Geometry check sheet. Reference: the model listing, model coordinates, mm. A direction names the side the tool comes from. Round coordinates to 2 decimals unless told otherwise and drop trailing zeros. Loops run counter-clockwise (first coordinate to the right, second up) from the corner with the lowest first, then second, coordinate; pieces in that order, holes last.
Autodesk Fusion 360 part; units mm, degrees
sketch "Sketch1" plane through (0, 0, 0) normal (0, 1, 0) x (1, 0, 0)
  line L0 (0, 0) -> (20.5, 0)
  line L1 (20.5, 0) -> (20.5, -10)
  line L2 (20.5, -10) -> (0, -10)
  line L3 (0, -10) -> (0, 0)
  line L4 (25.25, 0) -> (-4.75, 0)
  line L5 (-4.75, 0) -> (-4.75, -10)
  line L6 (-4.75, -10) -> (25.25, -10)
  line L7 (25.25, -10) -> (25.25, 0)
  line L8 (25.25, 0) -> (-4.75, -10) construction
  line L9 (-4.75, 0) -> (25.25, -10) construction
  line L10 (-4.75, 0) -> (-4.75, 6)
  line L11 (-4.75, 6) -> (25.25, 6)
  line L12 (25.25, 0) -> (25.25, 6)
  line L13 (-4.75, 6) -> (-4.75, 10)
  line L14 (-4.75, 10) -> (25.25, 10)
  line L15 (25.25, 10) -> (25.25, 6)
  line L16 (10.25, 0) -> (10.25, 10) construction
  line L17 (10.25, 0) -> (10.25, 2) construction
  line L18 (10.25, 2) -> (17.25, 2) construction
  line L19 (17.25, 2) -> (10.25, 2) construction
  line L20 (10.25, 2) -> (3.25, 2) construction
  circle A0 centre (3.25, 4) radius 2
  circle A1 centre (17.25, 4) radius 2
  point P0 (10.25, -5)
  dimension "d1" = 20.5
  dimension "d2" = 10
  dimension "d3" = 30
  dimension "d4" = 10
  dimension "d5" = 6
  dimension "d6" = 2
  dimension "d7" = 7
  dimension "d8" = 7
  dimension "d9" = 4
extrude "Extrude1" add sketch "Sketch1" along normal blind 40 contours L0 L4 L10 L11 L12 | L3 L4 L5 L6 | L1 L4 L6 L7 | L11 L13 L14 L15
sketch "Boceto3" plane through (25.25, 0, 0) normal (1, 0, 0) x (0, 1, 0)
  line L0 (0, 10) -> (0, -10)
  line L1 (0, -10) -> (40, -10)
  line L2 (40, -10) -> (40, 10)
  line L3 (40, 10) -> (0, 10)
  line L4 (0, -10) -> (0, -6)
  circle A0 centre (28, -6) radius 2
  circle A1 centre (8, -6) radius 2
  dimension "d12" = 4
  dimension "d13" = 4
  dimension "d14" = 4
delete_face "SuprimirCaras1" 1 faces at (5.2401, 13.3333, -3.8009)
delete_face "SuprimirCaras2" 1 faces at (19.2401, 13.3333, -3.8009)
hole "Agujero1" at (25.25, 8, -6) at (25.25, 28, -6) direction (-1, 0, 0) diameter 4 depth 36 tip angle 180
1) Mould release check, pull along X, two halves, no side actions. Record for faces 1 (the face through (0, 20, 5)), 2 (the face through (10.04, 6.648, -4.526)), 3 (the face through (25.25, 20, 0)): +X half, -X half, draft (parallel to the pull), parting line (faces both ways), or undercut.
Report:
face 1: undercut
face 2: draft
face 3: +X half
2) Access from +Z, -Z, +X, -X, +Y, -Y to the whole of each face (thin tool, end or side, straight path). Record for faces 4 (the face through (10, 20, 0)), 5 (the face through (10, 20, -10)).
Report:
face 4: +Z, +Y, -Y
face 5: -Z, +X, -X, +Y, -Y
3) Sectioned sample at B-B, the plane z = -6. Record the cut outline in (x, y), then the cut area to 3 significant figures.
Report:
outline: (-4.75, 0) - (25.25, 0) - (25.25, 6) - (-4.75, 6) - close; (-4.75, 10) - (25.25, 10) - (25.25, 26) - (-4.75, 26) - close; (-4.75, 30) - (25.25, 30) - (25.25, 40) - (-4.75, 40) - close
area: 960 mm2
4) Sectioned sample at D-D, the plane x = 21.5. Record the cut outline in (y, z).
Report:
outline: (0, -10) - (40, -10) - (40, 10) - (0, 10) - close; hole circle Ø4 at (8, -6); hole circle Ø4 at (28, -6)
5) Sectioned sample at A-A, the plane z = 2. Record the cut outline in (x, y).
Report:
outline: (-4.75, 0) - (0, 0) - (0, 40) - (-4.75, 40) - close; (20.5, 0) - (25.25, 0) - (25.25, 40) - (20.5, 40) - close
6) Gauge pin test, flat ends, axial feed: pin 1 (5 mm diameter, centred on x = 16.5, y = 21.5, fed in from +Z); pin 2 (4.5 mm diameter, centred on y = 8, z = -6, fed in from -X). Record the tip position at first contact, or that the pin passes through.
Report:
pin 1: stops at z = 0
pin 2: stops at x = -4.75
7) Scan lines: line 1 along Y through (x, z) = (6.5, -6); line 2 along X through (y, z) = (30, 8); line 3 along Z through (x, y) = (17.75, 28). Record each from-to range of solid material in increasing order.
Report:
line 1: y = 0 to 6, 10 to 26, 30 to 40
line 2: x = -4.75 to 0, 20.5 to 25.25
line 3: z = -10 to -8, -4 to 0
8) Sectioned sample at C-C, the plane y = 8. Record the cut outline in (x, z).
Report:
outline: (-4.75, -10) - (25.25, -10) - (25.25, -8) - (-4.75, -8) - close; (-4.75, -4) - (25.25, -4) - (25.25, 10) - (20.5, 10) - (20.5, 0) - (0, 0) - (0, 10) - (-4.75, 10) - close
